Verification items for the finished model (mm, model axes). Face numbers are marked on the shaded views. Coordinates: 2 decimals unless noted, no trailing zeros. Order: outer loops, then holes, each group sorted by start corner. A loop starts at its lowest first (then second) coordinate and runs counter-clockwise, first axis right, second up. Notation, with made-up numbers: (-25.75, -2.5) -> (-19.75, -2.5) arc R13 ccw to (-19.75, 17.5) -> close; hole circle Ø8 at (39, 48.25). An arc over 180 degrees is marked (long way). Write each question's results on one line, items separated by ' | '. Start each with the question number.
(1) Cross-section at A-A on z = 6. Enter the section's corners in (x, y), and give its area (3 significant figures).
(2) Thickness scan on probe 1 along Y at (x, z) = (0, 5); probe 2 along X at (y, z) = (0.75, 7.5); probe 3 along Y at (x, z) = (0.75, 5). Record the ranges inside material, lowest first. Write a range as [from, to].
(3) Go/stop test with flat-tipped pins: pin 1 (6 mm diameter, centred on x = 4, y = -5, fed in from -Z); pin 2 (3 mm diameter, centred on x = -7, z = 3.5, fed in from +Y); pin 3 (4 mm diameter, centred on y = -3.5, z = 7, fed in from -X). Record where each tip stops, or that it passes through.
(4) Draft check along Y on the marked faces 1, 2 and 3. Enter one of: +Y half, -Y half, draft (parallel to the pull), parting line (faces both ways), or undercut.
Solid Edge part; units mm, degrees
sketch "Sketch1" plane through (0, 0, 0) normal (0, 0, 1) x (1, 0, 0)
  line L0 (-4.6188, -8) -> (4.6188, -8)
  line L1 (4.6188, -8) -> (9.2376, 0)
  line L2 (9.2376, 0) -> (4.6188, 8)
  line L3 (4.6188, 8) -> (-4.6188, 8)
  line L4 (-4.6188, 8) -> (-9.2376, 0)
  line L5 (-9.2376, 0) -> (-4.6188, -8)
extrude "Protrusion1" add sketch "Sketch1" along normal blind 8.3
sketch "Sketch2" plane through (0, 0, 0) normal (0, -1, 0) x (1, 0, 0)
  line L0 (-8, 8.3) -> (-9.2376, 7.5855)
revolve "RevolvedCutout1" cut sketch "Sketch2" angle 360 about axis through (0, 0, 57.15) along (0, 0, -1) material side at (-8.6438, 0, 7.9861)
sketch "Sketch3" plane through (0, 0, 0) normal (0, -1, 0) x (1, 0, 0)
  line L0 (-8, 0) -> (-9.2376, 0.7145)
revolve "RevolvedCutout2" cut sketch "Sketch3" angle 360 about axis through (0, 0, 57.15) along (0, 0, -1) material side at (-8.6438, 0, 0.3139)
sketch "Sketch4" plane through (0, 0, 0) normal (0, 0, 1) x (1, 0, 0)
  circle A0 centre (0, 0) radius 4.188
extrude "Cutout1" cut sketch "Sketch4" along normal through all and the other way through all
chamfer "Chamfer1" distance 0.75 angle 45 2 edges at (-4.188, 0, 8.3) (-4.188, 0, 0)
cosmetic_thread "Thread1"
properties material "Steel"
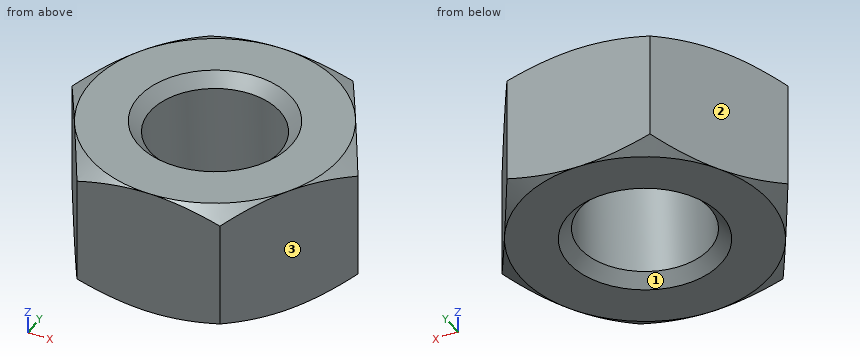
Results are:
1) outline: (-9.24, 0) -> (-4.62, -8) -> (4.62, -8) -> (9.24, 0) -> (4.62, 8) -> (-4.62, 8) -> close; hole circle Ø8.38 at (0, 0) | area: 167 mm2
2) probe 1: y = [-8, -4.19], [4.19, 8] | probe 2: x = [-8.8, -4.12], [4.12, 8.8] | probe 3: y = [-8, -4.12], [4.12, 8]
3) pin 1: stops at z = 0 | pin 2: stops at y = 6.47 | pin 3: stops at x = -8.37
4) face 1: undercut | face 2: +Y half | face 3: -Y half
